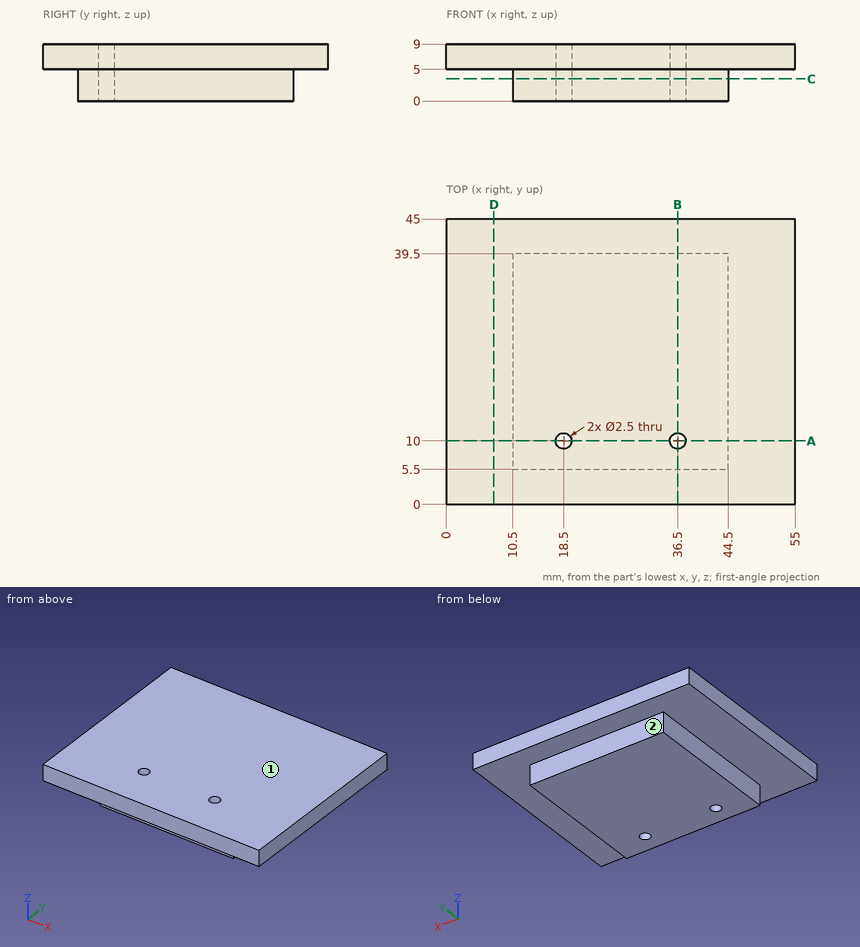
The figure shows three views and two pictorial views of one solid part (mm, origin at its lowest corner). Answer the questions. A direction names the side the tool comes from. Coordinates: 2 decimals unless noted, no trailing zeros. Order: outer loops, then holes, each group sorted by start corner. A loop starts at its lowest first (then second) coordinate and runs counter-clockwise, first axis right, second up. Notation, with made-up numbers: M 67,42 L 94,42 A35 ccw 94,80 Z; hole C 49,-12.5 d1. An arc over 180 degrees is marked long. Use CSV: the item, a comma, the result in double quotes.
1) Section A-A on y = 10 is taken. Write down the section's boundary in (x, z).
Worked out:
outline,"M 0,5 L 10.5,5 L 10.5,0 L 17.25,0 L 17.25,9 L 0,9 Z; M 19.75,0 L 35.25,0 L 35.25,9 L 19.75,9 Z; M 37.75,0 L 44.5,0 L 44.5,5 L 55,5 L 55,9 L 37.75,9 Z"
2) Section B-B on x = 36.5 is taken. Write down the section's boundary in (y, z), plus the area to 4 significant figures.
Worked out:
outline,"M 0,5 L 5.5,5 L 5.5,0 L 8.75,0 L 8.75,9 L 0,9 Z; M 11.25,0 L 39.5,0 L 39.5,5 L 45,5 L 45,9 L 11.25,9 Z"
area,"327.5 mm^2"
3) For the marked faces 1 and 2, determine the directions among +Z, -Z, +X, -X, +Y, -Y from which every point of the face is accessible in a straight line to the end or side of a thin tool.
Worked out:
face 1,"+Z, +X, -X, +Y, -Y"
face 2,"-Z, +X, -X, +Y"
4) Consider line 1 (X direction, y = 10, z = 5.75); line 2 (X direction, y = 9, z = 1.25); line 3 (Z direction, x = 5, y = 18). Determine where each line is inside the solid, lowest interval first. Write a range as [from, to].
Worked out:
line 1,"x = [0, 17.25], [19.75, 35.25], [37.75, 55]"
line 2,"x = [10.5, 17.75], [19.25, 35.75], [37.25, 44.5]"
line 3,"z = [5, 9]"
5) Section C-C on z = 3.5 is taken. Write down the section's boundary in (x, y).
Worked out:
outline,"M 10.5,5.5 L 44.5,5.5 L 44.5,39.5 L 10.5,39.5 Z; hole C 18.5,10 d2.5; hole C 36.5,10 d2.5"
6) Flat-ended cylindrical pins translate along their axes: pin 1 Ø2 at (y, z) = (31.5, 1) entering from +X; pin 2 Ø1.5 at (x, z) = (34, 2.5) entering from -Y; pin 3 Ø2.5 at (y, z) = (22.5, 2.5) entering from -X. Find the tip coordinate at first contact, or state that the pin passes through.
Worked out:
pin 1,"stops at x = 44.5"
pin 2,"stops at y = 5.5"
pin 3,"stops at x = 10.5"
7) Section D-D on x = 7.5 is taken. Write down the section's boundary in (y, z), plus the area to 3 significant figures.
Worked out:
outline,"M 0,5 L 45,5 L 45,9 L 0,9 Z"
area,"180 mm^2"
